Read the model definition and answer for the solid it produces. Units are mm, in the model's axes. Coordinates: 2 decimals unless noted, no trailing zeros. Order: outer loops, then holes, each group sorted by start corner. A loop starts at its lowest first (then second) coordinate and runs counter-clockwise, first axis right, second up. Notation, with made-up numbers: (11, 49) -> (18, 49) arc R32 ccw to (18, 77) -> close; hole circle Ø9 at (81, 52). An arc over 180 degrees is marked (long way). Use CSV: the item, a comma, the result in double quotes.
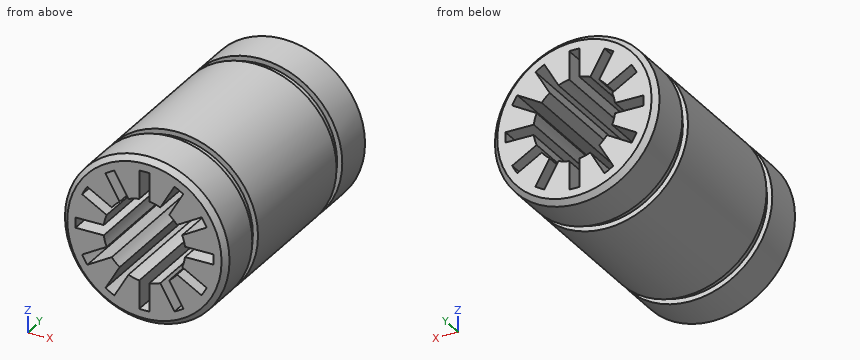
```python
from build123d import *

# Parameters (mm, degrees)
CHANFREIN1_SIZE         = 0.5
ENL_V_MAT_EXTRU_1_DEPTH = 25.8


with BuildPart() as part:
    # Esquisse2 → Révolution1 (revolve)
    with BuildSketch(Plane.XY):
        Polygon((0, 12.4), (-8.03826441, 12.4), (-8.03826441, 7.9), (-7.53826441, 7.9), (-7.53826441, 6.9), (-8.03826441, 6.9), (-8.03826441, -6.9), (-7.53826441, -6.9), (-7.53826441, -7.9), (-8.03826441, -7.9), (-8.03826441, -12.4), (0, -12.4), align=None)
    revolve(axis=Axis((0, 0, 0), (0, -1, 0)))

    # Chanfrein1
    chanfrein1_edges = [part.edges().sort_by_distance(p)[0] for p in [
        (8.03826441, 12.4, 0),
        (8.03826441, -12.4, 0),
    ]]
    chamfer(chanfrein1_edges, length=CHANFREIN1_SIZE)

    # Esquisse3 → Enlèv. mat.-Extru.1 (cut, through all)
    with BuildSketch(Plane(origin=(0, 12.4, 0), x_dir=(1, 0, 0), z_dir=(0, 1, 0))):
        with BuildLine():
            Line((-0.5, 6.731456009), (-0.5, 3.968626967))
            ThreePointArc((-0.5, 3.968626967), (-1.03527618, 3.863703305), (-1.551300781, 3.686931771))
            Line((-1.551300781, 3.686931771), (-2.932715303, 6.079611908))
            ThreePointArc((-2.932715303, 6.079611908), (-3.375, 5.845671476), (-3.798740706, 5.579611908))
            Line((-3.798740706, 5.579611908), (-2.417326185, 3.186931771))
            ThreePointArc((-2.417326185, 3.186931771), (-2.828427125, 2.828427125), (-3.186931771, 2.417326185))
            Line((-3.186931771, 2.417326185), (-5.579611908, 3.798740706))
            ThreePointArc((-5.579611908, 3.798740706), (-5.845671476, 3.375), (-6.079611908, 2.932715303))
            Line((-6.079611908, 2.932715303), (-3.686931771, 1.551300781))
            ThreePointArc((-3.686931771, 1.551300781), (-3.863703305, 1.03527618), (-3.968626967, 0.5))
            Line((-3.968626967, 0.5), (-6.731456009, 0.5))
            ThreePointArc((-6.731456009, 0.5), (-6.75, 0), (-6.731456009, -0.5))
            Line((-6.731456009, -0.5), (-3.968626967, -0.5))
            ThreePointArc((-3.968626967, -0.5), (-3.863703305, -1.03527618), (-3.686931771, -1.551300781))
            Line((-3.686931771, -1.551300781), (-6.079611908, -2.932715303))
            ThreePointArc((-6.079611908, -2.932715303), (-5.845671476, -3.375), (-5.579611908, -3.798740706))
            Line((-5.579611908, -3.798740706), (-3.186931771, -2.417326185))
            ThreePointArc((-3.186931771, -2.417326185), (-2.828427125, -2.828427125), (-2.417326185, -3.186931771))
            Line((-2.417326185, -3.186931771), (-3.798740706, -5.579611908))
            ThreePointArc((-3.798740706, -5.579611908), (-3.375, -5.845671476), (-2.932715303, -6.079611908))
            Line((-2.932715303, -6.079611908), (-1.551300781, -3.686931771))
            ThreePointArc((-1.551300781, -3.686931771), (-1.03527618, -3.863703305), (-0.5, -3.968626967))
            Line((-0.5, -3.968626967), (-0.5, -6.731456009))
            ThreePointArc((-0.5, -6.731456009), (0, -6.75), (0.5, -6.731456009))
            Line((0.5, -6.731456009), (0.5, -3.968626967))
            ThreePointArc((0.5, -3.968626967), (1.03527618, -3.863703305), (1.551300781, -3.686931771))
            Line((1.551300781, -3.686931771), (2.932715303, -6.079611908))
            ThreePointArc((2.932715303, -6.079611908), (3.375, -5.845671476), (3.798740706, -5.579611908))
            Line((3.798740706, -5.579611908), (2.417326185, -3.186931771))
            ThreePointArc((2.417326185, -3.186931771), (2.828427125, -2.828427125), (3.186931771, -2.417326185))
            Line((3.186931771, -2.417326185), (5.579611908, -3.798740706))
            ThreePointArc((5.579611908, -3.798740706), (5.845671476, -3.375), (6.079611908, -2.932715303))
            Line((6.079611908, -2.932715303), (3.686931771, -1.551300781))
            ThreePointArc((3.686931771, -1.551300781), (3.863703305, -1.03527618), (3.968626967, -0.5))
            Line((3.968626967, -0.5), (6.731456009, -0.5))
            ThreePointArc((6.731456009, -0.5), (6.75, 0), (6.731456009, 0.5))
            Line((6.731456009, 0.5), (3.968626967, 0.5))
            ThreePointArc((3.968626967, 0.5), (3.863703305, 1.03527618), (3.686931771, 1.551300781))
            Line((3.686931771, 1.551300781), (6.079611908, 2.932715303))
            ThreePointArc((6.079611908, 2.932715303), (5.845671476, 3.375), (5.579611908, 3.798740706))
            Line((5.579611908, 3.798740706), (3.186931771, 2.417326185))
            ThreePointArc((3.186931771, 2.417326185), (2.828427125, 2.828427125), (2.417326185, 3.186931771))
            Line((2.417326185, 3.186931771), (3.798740706, 5.579611908))
            ThreePointArc((3.798740706, 5.579611908), (3.375, 5.845671476), (2.932715303, 6.079611908))
            Line((2.932715303, 6.079611908), (1.551300781, 3.686931771))
            ThreePointArc((1.551300781, 3.686931771), (1.03527618, 3.863703305), (0.5, 3.968626967))
            Line((0.5, 3.968626967), (0.5, 6.731456009))
            ThreePointArc((0.5, 6.731456009), (0, 6.75), (-0.5, 6.731456009))
        make_face()
    extrude(amount=-ENL_V_MAT_EXTRU_1_DEPTH, mode=Mode.SUBTRACT)


solid = part.part
```
Item 1: Find section C-C, the plane x = 4.25. Give the number of separate pieces and of enclosed holes in the cut face, then the cut area to 3 significant figures.
Return value:
separate pieces,"4"
enclosed holes,"0"
area,"253 mm^2"
Item 2: Each of these flat-tipped pins is pushed along its axis until it touches: P1, Ø2, axis at y = -5.5, z = 5, coming from the -X side; P2, Ø1, axis at x = -3.5, y = 7, coming from the -Z side; P3, Ø3, axis at x = 4.5, y = 7.5, coming from the -Z side. Where does it stop, or does it pass through?
Return value:
P1,"stops at x = -6.97"
P2,"stops at z = -7.45"
P3,"stops at z = -7.44"
Item 3: Straight lines are drawn through the part: line 1 along Z through (x, y) = (0.25, -0.25); line 2 along X through (y, z) = (-5.25, 5); line 3 along X through (y, z) = (7.25, 5). For each, find the intervals that lie inside material, in ascending order.
Return value:
line 1,"z = -8.03 to -6.75, 6.75 to 8.03"
line 2,"x = -6.29 to -3.46, -2.31 to -0.5, 0.5 to 2.31, 3.46 to 6.29"
line 3,"x = -5.64 to -3.46, -2.31 to -0.5, 0.5 to 2.31, 3.46 to 5.64"
Item 4: Find section B-B, the plane x = 0. Give the vertices of the cut face in (y, z).
Return value:
outline,"(-12.4, -7.54) -> (-11.9, -8.04) -> (-7.9, -8.04) -> (-7.9, -7.54) -> (-6.9, -7.54) -> (-6.9, -8.04) -> (6.9, -8.04) -> (6.9, -7.54) -> (7.9, -7.54) -> (7.9, -8.04) -> (11.9, -8.04) -> (12.4, -7.54) -> (12.4, -6.75) -> (-12.4, -6.75) -> close; (-12.4, 6.75) -> (12.4, 6.75) -> (12.4, 7.54) -> (11.9, 8.04) -> (7.9, 8.04) -> (7.9, 7.54) -> (6.9, 7.54) -> (6.9, 8.04) -> (-6.9, 8.04) -> (-6.9, 7.54) -> (-7.9, 7.54) -> (-7.9, 8.04) -> (-11.9, 8.04) -> (-12.4, 7.54) -> close"
Item 5: Find section A-A, the plane z = 0. Give the vertices of the cut face in (x, y).
Return value:
outline,"(-8.04, -11.9) -> (-7.54, -12.4) -> (-6.75, -12.4) -> (-6.75, 12.4) -> (-7.54, 12.4) -> (-8.04, 11.9) -> (-8.04, 7.9) -> (-7.54, 7.9) -> (-7.54, 6.9) -> (-8.04, 6.9) -> (-8.04, -6.9) -> (-7.54, -6.9) -> (-7.54, -7.9) -> (-8.04, -7.9) -> close; (6.75, -12.4) -> (7.54, -12.4) -> (8.04, -11.9) -> (8.04, -7.9) -> (7.54, -7.9) -> (7.54, -6.9) -> (8.04, -6.9) -> (8.04, 6.9) -> (7.54, 6.9) -> (7.54, 7.9) -> (8.04, 7.9) -> (8.04, 11.9) -> (7.54, 12.4) -> (6.75, 12.4) -> close"
